Drawing for the job (mm, zero at the part's lowest x, y, z). Coordinates: 2 decimals unless noted, no trailing zeros. Loops run counter-clockwise (first coordinate to the right, second up) from the corner with the lowest first, then second, coordinate; pieces in that order, holes last. Notation, with made-up numbers: (-26.75, -18.75) - (-3.75, -18.75) arc R34 cw to (-3.75, 12.25) - close; hole circle Ø1 at (43.5, -6.75). An arc over 180 degrees is marked (long way). One line per item, written item: value.
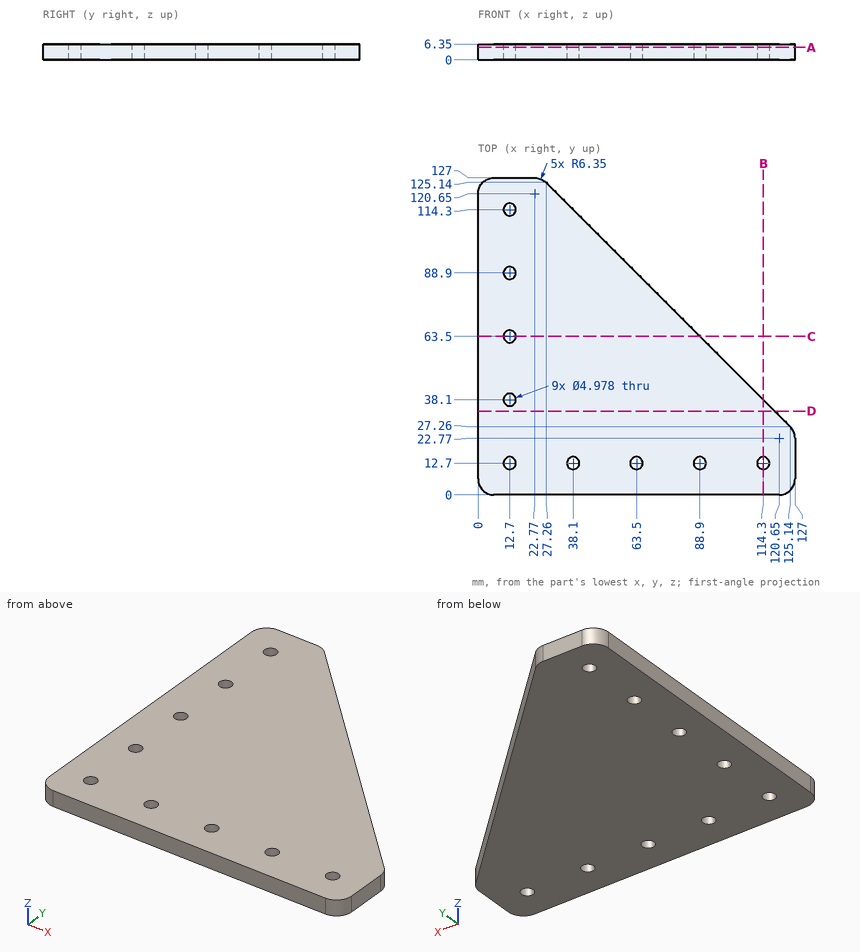
Item 1: Cut at D-D, the plane y = 33.5. Write the cut outline in (x, z).
Check result:
outline: (0, 0) - (118.9, 0) - (118.9, 6.35) - (0, 6.35) - close
Item 2: Drop flat-ended pins along their axis: P1, Ø6.5, axis at x = 12.7, y = 114.3, coming from the -Z side; P2, Ø4, axis at x = 114.3, y = 12.7, coming from the +Z side; P3, Ø1.5, axis at x = 91, z = 3.5, coming from the +Y side; P4, Ø1, axis at y = 103, z = 1, coming from the +X side. Give the stop position or say it passes through.
Check result:
P1: stops at z = 0
P2: passes through
P3: stops at y = 62.15
P4: stops at x = 49.9
Item 3: Probe probe 1 along Y at (x, z) = (12.7, 3.5); probe 2 along X at (y, z) = (13, 2.75); probe 3 along Y at (x, z) = (114.3, 5.25). List the from-to ranges inside material, lowest first. Write a range as from..to.
Check result:
probe 1: y = 0..10.21, 15.19..35.61, 40.59..61.01, 65.99..86.41, 91.39..111.81, 116.79..127
probe 2: x = 0..10.23, 15.17..35.63, 40.57..61.03, 65.97..86.43, 91.37..111.83, 116.77..127
probe 3: y = 0..10.21, 15.19..38.1
Item 4: Cut at A-A, the plane z = 5. Give the number of separate pieces and of enclosed holes in the cut face, then the cut area to 3 significant figures.
Check result:
separate pieces: 1
enclosed holes: 9
area: 10,800 mm^2
Item 5: Cut at C-C, the plane y = 63.5. Write the cut outline in (x, z).
Check result:
outline: (0, 0) - (10.21, 0) - (10.21, 6.35) - (0, 6.35) - close; (15.19, 0) - (88.9, 0) - (88.9, 6.35) - (15.19, 6.35) - close
Item 6: Cut at B-B, the plane x = 114.3. Write the cut outline in (y, z).
Check result:
outline: (0, 0) - (10.21, 0) - (10.21, 6.35) - (0, 6.35) - close; (15.19, 0) - (38.1, 0) - (38.1, 6.35) - (15.19, 6.35) - close
